Autodesk Inventor part; units mm, degrees
ref_plane "YZ Plane" through (0, 0, 0) normal (1, 0, 0) x (0, 1, 0)
ref_plane "XZ Plane" through (0, 0, 0) normal (0, 1, 0) x (-1, 0, 0)
ref_plane "XY Plane" through (0, 0, 0) normal (0, 0, 1) x (1, 0, 0)
sketch "Sketch1" plane through (0, 0, 0) normal (0, 0, 1) x (1, 0, 0)
  line L0 (45.72, 0) -> (45.72, 60.96)
  line L1 (45.72, 60.96) -> (-45.72, 60.96)
  line L2 (-45.72, 60.96) -> (-45.72, 9.301)
  line L3 (-45.72, 5.08) -> (-50.8, 5.08)
  line L4 (-50.8, 5.08) -> (-50.8, 15.24)
  line L5 (-50.8, 15.24) -> (-45.72, 15.24)
  line L6 (-45.72, 15.24) -> (-45.72, 5.08)
  line L7 (-45.72, 25.4) -> (-50.8, 25.4)
  line L8 (-50.8, 25.4) -> (-50.8, 35.56)
  line L9 (-50.8, 35.56) -> (-45.72, 35.56)
  line L10 (-45.72, 35.56) -> (-45.72, 25.4)
  line L11 (-45.72, 45.72) -> (-50.8, 45.72)
  line L12 (-50.8, 45.72) -> (-50.8, 55.88)
  line L13 (-50.8, 55.88) -> (-45.72, 55.88)
  line L14 (-45.72, 55.88) -> (-45.72, 45.72)
  line L15 (0, 60.96) -> (0, 0) construction
  line L16 (45.72, 60.96) -> (45.72, 0)
  line L17 (45.72, 5.08) -> (50.8, 5.08)
  line L18 (50.8, 5.08) -> (50.8, 15.24)
  line L19 (50.8, 15.24) -> (45.72, 15.24)
  line L20 (45.72, 15.24) -> (45.72, 5.08)
  line L21 (45.72, 25.4) -> (50.8, 25.4)
  line L22 (50.8, 25.4) -> (50.8, 35.56)
  line L23 (50.8, 35.56) -> (45.72, 35.56)
  line L24 (45.72, 35.56) -> (45.72, 25.4)
  line L25 (45.72, 45.72) -> (50.8, 45.72)
  line L26 (50.8, 45.72) -> (50.8, 55.88)
  line L27 (50.8, 55.88) -> (45.72, 55.88)
  line L28 (45.72, 55.88) -> (45.72, 45.72)
  line L29 (-45.72, 5.08) -> (-45.72, 0)
  line L30 (-45.72, 0) -> (45.72, 0)
  line L31 (45.72, 60.96) -> (-45.72, 60.96)
  line L32 (-45.72, 60.96) -> (-45.72, 0)
  line L33 (-45.72, 0) -> (45.72, 0)
  line L34 (45.72, 0) -> (45.72, 60.96)
  dimension "d0" = 91.44
  dimension "d2" = 10.16
  dimension "d3" = 5.08
  dimension "d7" = 20.32
  dimension "d14" = 5.08
  dimension "d15" = 60.96
extrude "Extrusion2" add sketch "Sketch1" along normal blind 5.08
sketch "Sketch2" plane through (0, 0, 0) normal (0, 0, -1) x (-1, 0, 0)
  circle A0 centre (-15.5, 5.5) radius 1.5
  circle A1 centre (15.5, 36.5) radius 1.5
  circle A2 centre (-15.5, 36.5) radius 1.5
  circle A3 centre (15.5, 5.5) radius 1.5
  line L0 (21, 3.175) -> (17.825, 0)
  line L1 (21, 38.825) -> (21, 3.175)
  line L2 (17.825, 42) -> (21, 38.825)
  line L3 (-17.825, 42) -> (17.825, 42)
  line L4 (-21, 38.825) -> (-17.825, 42)
  line L5 (-21, 3.175) -> (-21, 38.825)
  line L6 (-17.825, 0) -> (-21, 3.175)
  line L7 (17.825, 0) -> (-17.825, 0)
  circle A4 centre (0, 21) radius 11
  circle A5 centre (0, 21) radius 2.25
  point P0 (0, 0)
extrude "Extrusion3" cut sketch "Sketch2" against normal blind 25.4 contours A0 | A1 | A2 | A3 | A4 | A5
sketch "Sketch4" plane through (0, 0, 5.08) normal (0, 0, 1) x (1, 0, 0)
  line L0 (0, 0) -> (0, 60.96) construction
  line L1 (45.72, 60.96) -> (-45.72, 60.96) construction
  line L2 (-30.48, 52.75) -> (-5.08, 52.75) construction
  line L3 (-30.48, 51.25) -> (-5.08, 51.25)
  line L4 (-5.08, 54.25) -> (-30.48, 54.25)
  arc A0 (-30.48, 54.25) -> (-30.48, 51.25) centre (-30.48, 52.75) ccw
  arc A1 (-5.08, 51.25) -> (-5.08, 54.25) centre (-5.08, 52.75) ccw
  line L5 (30.48, 52.75) -> (5.08, 52.75) construction
  line L6 (30.48, 51.25) -> (5.08, 51.25)
  line L7 (5.08, 54.25) -> (30.48, 54.25)
  arc A2 (30.48, 51.25) -> (30.48, 54.25) centre (30.48, 52.75) ccw
  arc A3 (5.08, 54.25) -> (5.08, 51.25) centre (5.08, 52.75) ccw
  circle A4 centre (0, 21) radius 11
  line L8 (-11, 21) -> (0, 21)
  point P0 (-17.78, 52.75)
  point P1 (17.78, 52.75)
  dimension "d25" = 3
  dimension "d26" = 25.4
  dimension "d28" = 17.78
  dimension "d31" = 31.75
extrude "Extrusion5" cut sketch "Sketch4" against normal blind 25.4 contours A0 L4 A1 L3 | L6 A3 L7 A2
sketch "Sketch5" plane through (0, 0, 5.08) normal (0, 0, 1) x (1, 0, 0)
  arc A0 (-5.08, 51.25) -> (-5.08, 54.25) centre (-5.08, 52.75) ccw
  line L0 (-5.08, 51.25) -> (-30.48, 51.25)
  arc A1 (-30.48, 54.25) -> (-30.48, 51.25) centre (-30.48, 52.75) ccw
  line L1 (-30.48, 54.25) -> (-5.08, 54.25)
  arc A2 (30.48, 51.25) -> (30.48, 54.25) centre (30.48, 52.75) ccw
  line L2 (30.48, 51.25) -> (5.08, 51.25)
  arc A3 (5.08, 54.25) -> (5.08, 51.25) centre (5.08, 52.75) ccw
  line L3 (5.08, 54.25) -> (30.48, 54.25)
  circle A4 centre (-15.5, 5.5) radius 1.5
  circle A5 centre (-15.5, 36.5) radius 1.5
  circle A6 centre (15.5, 5.5) radius 1.5
  circle A7 centre (15.5, 36.5) radius 1.5
  circle A8 centre (0, 21) radius 11
  line L4 (50.8, 25.4) -> (50.8, 35.56)
  line L5 (50.8, 35.56) -> (45.72, 35.56)
  line L6 (45.72, 35.56) -> (45.72, 45.72)
  line L7 (45.72, 45.72) -> (50.8, 45.72)
  line L8 (50.8, 45.72) -> (50.8, 55.88)
  line L9 (50.8, 55.88) -> (45.72, 55.88)
  line L10 (45.72, 55.88) -> (45.72, 60.96)
  line L11 (45.72, 60.96) -> (-45.72, 60.96)
  line L12 (-45.72, 60.96) -> (-45.72, 55.88)
  line L13 (-45.72, 55.88) -> (-50.8, 55.88)
  line L14 (-50.8, 55.88) -> (-50.8, 45.72)
  line L15 (-50.8, 45.72) -> (-45.72, 45.72)
  line L16 (-45.72, 45.72) -> (-45.72, 35.56)
  line L17 (-45.72, 35.56) -> (-50.8, 35.56)
  line L18 (-50.8, 35.56) -> (-50.8, 25.4)
  line L19 (-50.8, 25.4) -> (-45.72, 25.4)
  line L20 (-45.72, 25.4) -> (-45.72, 15.24)
  line L21 (-45.72, 15.24) -> (-50.8, 15.24)
  line L22 (-50.8, 15.24) -> (-50.8, 5.08)
  line L23 (-50.8, 5.08) -> (-45.72, 5.08)
  line L24 (-45.72, 5.08) -> (-45.72, 0)
  line L25 (-45.72, 0) -> (45.72, 0)
  line L26 (45.72, 0) -> (45.72, 5.08)
  line L27 (45.72, 5.08) -> (50.8, 5.08)
  line L28 (50.8, 5.08) -> (50.8, 15.24)
  line L29 (50.8, 15.24) -> (45.72, 15.24)
  line L30 (45.72, 15.24) -> (45.72, 25.4)
  line L31 (45.72, 25.4) -> (50.8, 25.4)
  point P0 (0, 0)
  dimension "d32" = 21
equation "\"d7\" = 2 * d2"
properties part number "VerticalSupport" material "Wood (Birch)"
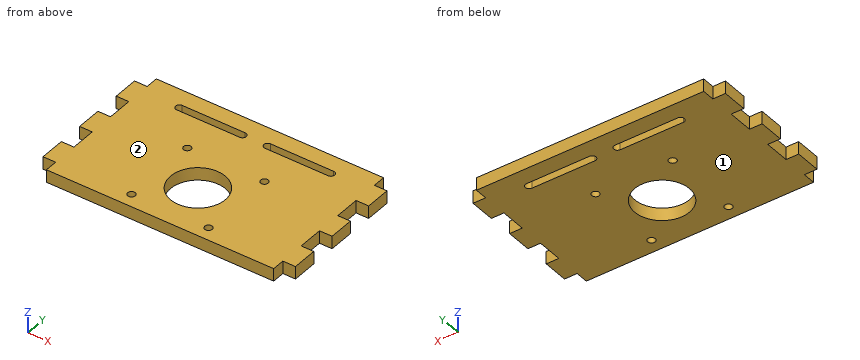
Could you check a few things on this model? Use its own coordinates, in mm. Face numbers are marked on the shaded views. Round coordinates to 2 decimals unless told otherwise and drop trailing zeros. Order: outer loops, then holes, each group sorted by start corner. A loop starts at its lowest first (then second) coordinate and runs counter-clockwise, first axis right, second up. Notation, with made-up numbers: M 70,33 L 129,33 A24 ccw 129,45 Z; hole C 4,-21 d9. An arc over 180 degrees is marked long. One line per item, written item: value.
(1) Imagine slicing it at B-B (y = 52.75). Write out the boundary of the cut face in (x, z), and give its area (3 significant figures).
Ans:
outline: M -50.8,0 L -31.98,0 L -31.98,5.08 L -50.8,5.08 Z; M -3.58,0 L 3.58,0 L 3.58,5.08 L -3.58,5.08 Z; M 31.98,0 L 50.8,0 L 50.8,5.08 L 31.98,5.08 Z
area: 228 mm^2
(2) Imagine slicing it at D-D (y = 21). Write out the boundary of the cut face in (x, z), and give its area (3 significant figures).
Ans:
outline: M -45.72,0 L -11,0 L -11,5.08 L -45.72,5.08 Z; M 11,0 L 45.72,0 L 45.72,5.08 L 11,5.08 Z
area: 353 mm^2
(3) If we mould it in two halves opening along Z, with no side actions, what happens to the marked faces 1 and 2? For each: released by +Z, released by -Z, zero draft, split by the parting line, or undercut.
Ans:
face 1: released by -Z
face 2: released by +Z
(4) I'm going to push flat-ended pins straight in: P1, Ø1.5, axis at y = 19.5, z = 1.5, coming from the +X side; P2, Ø3, axis at x = -34.5, y = 54.5, coming from the -Z side; P3, Ø1.5, axis at x = 48, z = 3.5, coming from the -Y side; P4, Ø1, axis at x = 9, y = 16, coming from the +Z side. Where does each tip first touch, or does it pass through?
Ans:
P1: stops at x = 45.72
P2: stops at z = 0
P3: stops at y = 5.08
P4: passes through
(5) I need wall thicknesses on line 1 along Y through (x, z) = (-15.5, 3.2); line 2 along X through (y, z) = (54, 4.8); line 3 along X through (y, z) = (28, 2.3). Which ranges of each line are inside material? Lowest first, please. Write a range as from..to.
Ans:
line 1: y = 0..4, 7..35, 38..51.25, 54.25..60.96
line 2: x = -50.8..-31.31, -4.25..4.25, 31.31..50.8
line 3: x = -50.8..-8.49, 8.49..50.8
(6) Imagine slicing it at C-C (x = -20.5). Write out the boundary of the cut face in (y, z).
Ans:
outline: M 0,0 L 51.25,0 L 51.25,5.08 L 0,5.08 Z; M 54.25,0 L 60.96,0 L 60.96,5.08 L 54.25,5.08 Z
(7) Imagine slicing it at A-A (x = 15.5). Write out the boundary of the cut face in (y, z), and give its area (3 significant figures).
Ans:
outline: M 0,0 L 4,0 L 4,5.08 L 0,5.08 Z; M 7,0 L 35,0 L 35,5.08 L 7,5.08 Z; M 38,0 L 51.25,0 L 51.25,5.08 L 38,5.08 Z; M 54.25,0 L 60.96,0 L 60.96,5.08 L 54.25,5.08 Z
area: 264 mm^2
